Geometry: final body of the model. Coordinates: model frame, mm. Give positions to 0.01 mm unless a question says otherwise; leave off trailing zeros. Write each loop counter-clockwise with the first axis right and the second up, starting at its lowest first coordinate (ties: lowest second). Pieces come first, ordered by that corner, then holes. Notation, with made-up numbers: (59, 38.25) -> (114, 38.25) arc R24 ccw to (114, 65.25) -> close; hole circle Ø9 at (-6.5, 8). An arc over 180 degrees is marked (long way). Answer as a JSON object with one key per item and string values.
from build123d import *

# Parameters (mm, degrees)
F0_W     = 94.914917
F0_H     = 35.086341
F1_DEPTH = 25.4
F2_R     = 5.08
F3_SIZE  = 5.08
F5_D     = 6.35


with BuildPart() as f1:
    # F0 (on Top) → F1 (new body)
    with BuildSketch(Plane.XY):
        with Locations((-40.582946, -17.54317)):
            Rectangle(F0_W, F0_H)
    extrude(amount=F1_DEPTH)

    # F2
    f2_edges = [f1.edges().sort_by_distance(p)[0] for p in [
        (-40.582946, -35.086341, 25.4),
        (6.874513, -17.543171, 25.4),
        (6.874513, -35.086341, 12.7),
        (-88.040404, -35.086341, 12.7),
    ]]
    fillet(f2_edges, radius=F2_R)

    # F3
    f3_edges = [f1.edges().sort_by_distance(p)[0] for p in [
        (-43.122946, 0, 25.4),
    ]]
    chamfer(f3_edges, length=F3_SIZE)

    # F5 (through all)
    with Locations(Plane(origin=(0, 0, 0), x_dir=(1, 0, 0), z_dir=(0, 0, -1))):
        with Locations((-79.811066, 26.63902)):
            Hole(F5_D / 2)


solid = f1.part
Q1. Cut plane D-D (y = -31.5). Return the cut outline in (x, z), and give its area (3 significant figures).
Values:
{"outline": "(-87.82, 0) -> (6.65, 0) -> (6.65, 20.32) arc R4.86 ccw to (1.79, 25.18) -> (-87.82, 25.18) -> close", "area": "2,370 mm²"}
Q2. Cut plane A-A (x = -79). Return the cut outline in (y, z).
Values:
{"outline": "(-35.09, 0) -> (-29.71, 0) -> (-29.71, 25.4) -> (-30.01, 25.4) arc R5.08 ccw to (-35.09, 20.32) -> close; (-23.57, 0) -> (0, 0) -> (0, 20.32) -> (-5.08, 25.4) -> (-23.57, 25.4) -> close"}
Q3. First-contact query: P1, Ø1.5, axis at x = -72, y = -23.5, coming from the -Z side. Flat tip, straight axial feed; report the tip coordinate or a pass-through.
Values:
{"P1": "z = 0"}
Q4. Mould query, pull axis X, two halves, no side actions, for faces 1 (the flat face through (-41, -35.086, 10)), 2 (the cylindrical face through (-77.29, -24.71, 12.88)), 3 (the cylindrical face through (5.4, -17.4, 23.9)). Classes: pulls with the +X half, pulls with the -X half, needs draft (parallel to the pull), parting line crosses it, or undercut.
Values:
{"face 1": "needs draft", "face 2": "undercut", "face 3": "pulls with the +X half"}
Q5. Material intervals for L1, parallel to Y at x = -49, z = 21.25; L2, parallel to Z at x = -53.5, y = -2; L3, parallel to Y at x = -82.5, z = 7, sorted ascending. Write a range as from..to.
Values:
{"L1": "-35..-0.93", "L2": "0..22.32", "L3": "-35.09..-28.33, -24.95..0"}
Q6. Cut plane B-B (z = 2.25). Return the cut outline in (x, y) (3 decimals).
Values:
{"outline": "(-88.04, -30.006) arc R5.08 ccw to (-82.96, -35.086) -> (1.795, -35.086) arc R5.08 ccw to (6.875, -30.006) -> (6.875, -5.08) -> (1.795, 0) -> (-88.04, 0) -> close; hole circle Ø6.35 at (-79.811, -26.639)"}
Q7. Cut plane C-C (x = -32.5). Return the cut outline in (y, z), and give its area (3 significant figures).
Values:
{"outline": "(-35.09, 0) -> (0, 0) -> (0, 20.32) -> (-5.08, 25.4) -> (-30.01, 25.4) arc R5.08 ccw to (-35.09, 20.32) -> close", "area": "873 mm²"}
